Autodesk Inventor part; units mm, degrees
ref_plane "YZ Plane" through (0, 0, 0) normal (1, 0, 0) x (0, 1, 0)
ref_plane "XZ Plane" through (0, 0, 0) normal (0, 1, 0) x (-1, 0, 0)
ref_plane "XY Plane" through (0, 0, 0) normal (0, 0, 1) x (1, 0, 0)
sketch "スケッチ1" plane through (0, 0, 0) normal (0, 1, 0) x (-1, 0, 0)
  line L0 (6, 15) -> (-6, 15)
  line L1 (-6, 15) -> (-6, -15)
  line L2 (-6, -15) -> (6, -15)
  line L3 (6, -15) -> (6, 15)
  line L4 (-6, 7) -> (-14, 7)
  line L5 (-14, 7) -> (-14, -7)
  line L6 (-14, -7) -> (-6, -7)
  line L7 (-6, -7) -> (-6, 7)
  circle A0 centre (0, 11) radius 1.5
  circle A1 centre (0, -11) radius 1.5
  point P0 (0, 0)
  dimension "d0" = 30
  dimension "d1" = 12
  dimension "d2" = 14
  dimension "d3" = 8
  dimension "d4" = 8
  dimension "d5" = 15
  dimension "d6" = 6
  dimension "d7" = 8
  dimension "d8" = 3
  dimension "d9" = 3
  dimension "d10" = 6
  dimension "d11" = 6
  dimension "d12" = 4
  dimension "d13" = 4
extrude "押し出し1" add sketch "スケッチ1" along normal blind 1.2 contours L3 L2 L1 L0
extrude "押し出し2" add sketch "スケッチ1" along normal blind 5 contours L1 L6 L5 L4
sketch "スケッチ2" plane through (0, 1.2, 0) normal (0, 1, 0) x (1, 0, 0)
  line L0 (-1, -2) -> (1, -2)
  line L1 (1, -2) -> (1, 2)
  line L2 (1, 2) -> (-1, 2)
  line L3 (-1, 2) -> (-1, -2)
  point P0 (0, 0)
  dimension "d18" = 2
  dimension "d19" = 4
  dimension "d20" = 2
  dimension "d21" = 1
extrude "押し出し3" add sketch "スケッチ2" along normal blind 1.2
properties part number "sensor"
Geometry: final body of the model. Coordinates: model frame, mm. A direction names the side the tool comes from. Coordinates: 2 decimals unless noted, no trailing zeros. Order: outer loops, then holes, each group sorted by start corner. A loop starts at its lowest first (then second) coordinate and runs counter-clockwise, first axis right, second up. Notation, with made-up numbers: (54, -21) -> (100, -21) arc R20 ccw to (100, -2) -> close; hole circle Ø5 at (-9.5, 48). An arc over 180 degrees is marked (long way). Answer in a Markdown table with one row per item.
Item 1: Section C-C on z = -5.5. Output: boundary loops of the cut face in (x, y).
Return value:
| item | result |
|---|---|
| outline | (-6, 0) -> (14, 0) -> (14, 5) -> (6, 5) -> (6, 1.2) -> (-6, 1.2) -> close |
Item 2: Section B-B on z = 11. Output: boundary loops of the cut face in (x, y), plus the area to 3 significant figures.
Return value:
| item | result |
|---|---|
| outline | (-6, 0) -> (-1.5, 0) -> (-1.5, 1.2) -> (-6, 1.2) -> close; (1.5, 0) -> (6, 0) -> (6, 1.2) -> (1.5, 1.2) -> close |
| area | 10.8 mm² |
Item 3: Access query for faces 1 (the flat face through (0, 2.4, 0)), 2 (the flat face through (0, 2, 2)), 3 (the flat face through (6, 1, 11)), 4 (the flat face through (1, 2, 0)), 5 (the flat face through (10, 2, -7)). Directions: +Z, -Z, +X, -X, +Y, -Y. A direction counts if a zero-diameter tool reaches every point of the face in a straight line with its end or side. Return the directions, or none.
Return value:
| item | result |
|---|---|
| face 1 | +Z, -Z, -X, +Y |
| face 2 | +Z, -X, +Y |
| face 3 | +Z, +X, +Y, -Y |
| face 4 | +Z, -Z, +Y |
| face 5 | -Z, +X, +Y, -Y |
Item 4: Draft query along X for faces 6 (the cylindrical face through (0.325, 0.592, 12.464)), 7 (the flat face through (-1, 2, 0)), 8 (the flat face through (10, 5, 0)). Return one class per face: released by +X, released by -X, zero draft, split by the parting line, or undercut.
Return value:
| item | result |
|---|---|
| face 6 | undercut |
| face 7 | released by -X |
| face 8 | zero draft |
Item 5: Contact query for flat-ended pins moving along their axis: P1, Ø3.5, axis at x = 2, z = 6.5, coming from the +Y side; P2, Ø1.5, axis at y = 2, z = -6.5, coming from the -X side; P3, Ø0.6, axis at y = 2, z = -0.5, coming from the -X side. Output: stop coordinate, or through.
Return value:
| item | result |
|---|---|
| P1 | stops at y = 1.2 |
| P2 | stops at x = 6 |
| P3 | stops at x = -1 |
Item 6: Ray query, L1, parallel to Z at x = 0, y = 0.9; L2, parallel to Z at x = 11, y = 3.25; L3, parallel to Y at x = 5.5, z = 7. Return the intervals inside material, ascending.
Return value:
| item | result |
|---|---|
| L1 | z = -15 to -12.5, -9.5 to 9.5, 12.5 to 15 |
| L2 | z = -7 to 7 |
| L3 | y = 0 to 1.2 |
Item 7: Section D-D on y = 3.7. Output: boundary loops of the cut face in (x, z).
Return value:
| item | result |
|---|---|
| outline | (6, -7) -> (14, -7) -> (14, 7) -> (6, 7) -> close |
Item 8: Section A-A on x = 0. Output: boundary loops of the cut face in (y, z).
Return value:
| item | result |
|---|---|
| outline | (0, -15) -> (1.2, -15) -> (1.2, -12.5) -> (0, -12.5) -> close; (0, -9.5) -> (1.2, -9.5) -> (1.2, -2) -> (2.4, -2) -> (2.4, 2) -> (1.2, 2) -> (1.2, 9.5) -> (0, 9.5) -> close; (0, 12.5) -> (1.2, 12.5) -> (1.2, 15) -> (0, 15) -> close |
